Geometry: final body of the model. Coordinates: model frame, mm. Face numbers are marked on the shaded views. A direction names the side the tool comes from. Coordinates: 2 decimals unless noted, no trailing zeros. Loops run counter-clockwise (first coordinate to the right, second up) from the corner with the lowest first, then second, coordinate; pieces in that order, holes last. Notation, with made-up numbers: (40, 35) - (78, 35) arc R10 ccw to (78, 51) - close; hole circle Ø3 at (18, -31). An arc over 180 degrees is marked (long way). Answer in a Markdown table with one row per item.
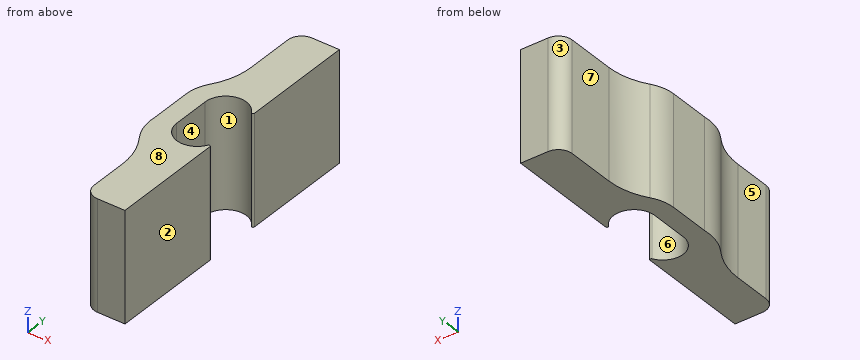
from build123d import *

# Parameters (mm, degrees)
F1_DEPTH = 8
F2_R     = 0.1
F3_R     = 1
F4_R     = 5


with BuildPart() as f1:
    # F0 (on Top) → F1 (new body)
    with BuildSketch(Plane.XY):
        with BuildLine():
            Line((0, -2.75), (0, 0))
            ThreePointArc((0, 0), (1.5, 1.5), (3, 0))
            Line((3, 0), (3, 9))
            Line((3, 9), (0, 9))
            Line((0, 9), (0, 2.4526771088))
            ThreePointArc((0, 2.4526771088), (-1.007800331, 1.4059027349), (-1.375, 0))
            Line((-1.375, 0), (-1.375, -3))
            ThreePointArc((-1.375, -3), (-1.1039614046, -4.7622217371), (0, -6.1622776602))
            Line((0, -6.1622776602), (0, -11.75))
            Line((0, -11.75), (3, -11.75))
            Line((3, -11.75), (3, -2.75))
            ThreePointArc((3, -2.75), (1.5, -4.25), (0, -2.75))
        make_face()
    extrude(amount=F1_DEPTH)

    # F2 (call 1 of 2: OpenCascade refuses the feature's edges together)
    f2_edges = [f1.edges().sort_by_distance(p)[0] for p in [
        (3, 0, 4),
    ]]
    fillet(f2_edges, radius=F2_R)

    # F2#2 (call 2 of 2)
    f2_2_edges = [f1.edges().sort_by_distance(p)[0] for p in [
        (3, -2.75, 4),
    ]]
    fillet(f2_2_edges, radius=F2_R)

    # F3
    f3_edges = [f1.edges().sort_by_distance(p)[0] for p in [
        (0, 9, 4),
        (0, -11.75, 4),
    ]]
    fillet(f3_edges, radius=F3_R)

    # F4
    f4_edges = [f1.edges().sort_by_distance(p)[0] for p in [
        (0, 2.452677, 4),
        (0, -6.162278, 4),
    ]]
    fillet(f4_edges, radius=F4_R)


solid = f1.part
(1) Cut plane B-B on x = 2.35. Output: boundary loops of the cut face in (y, z).
Verdict:
| item | result |
|---|---|
| outline | (-11.75, 0) - (-3.99, 0) - (-3.99, 8) - (-11.75, 8) - close; (1.24, 0) - (9, 0) - (9, 8) - (1.24, 8) - close |
(2) Access query for the marked faces 4, 5, 6, 7 and 8. Directions: +Z, -Z, +X, -X, +Y, -Y. A direction counts if a zero-diameter tool reaches every point of the face in a straight line with its end or side. Return the directions, or none.
Verdict:
| item | result |
|---|---|
| face 4 | +Z, -Z, +X |
| face 5 | +Z, -Z, -X, -Y |
| face 6 | +Z, -Z |
| face 7 | +Z, -Z, -X, +Y |
| face 8 | +Z, +X, -X, +Y, -Y |
(3) Ray query, probe 1 along X at (y, z) = (-1.75, 5.75) (3 decimals); probe 2 along Y at (x, z) = (1.85, 5); probe 3 along X at (y, z) = (5, 2.5). Return the intervals inside material, ascending.
Verdict:
| item | result |
|---|---|
| probe 1 | x = -1.375 to 0 |
| probe 2 | y = -11.75 to -4.21, 1.46 to 9 |
| probe 3 | x = 0 to 3 |
(4) Cut plane C-C on y = 6.75. Output: boundary loops of the cut face in (x, z), then the cut area to 3 significant figures.
Verdict:
| item | result |
|---|---|
| outline | (0, 0) - (3, 0) - (3, 8) - (0, 8) - close |
| area | 24.0 mm² |
(5) Pull-direction query (X, two-part tool) for the marked faces 1, 2 and 3; classes: pulls with the +X half, pulls with the -X half, needs draft (parallel to the pull), parting line crosses it, or undercut.
Verdict:
| item | result |
|---|---|
| face 1 | undercut |
| face 2 | pulls with the +X half |
| face 3 | pulls with the -X half |
(6) Cut plane D-D on x = -0.25. Output: boundary loops of the cut face in (y, z).
Verdict:
| item | result |
|---|---|
| outline | (-6.47, 0) - (2.88, 0) - (2.88, 8) - (-6.47, 8) - close |
(7) Cut plane A-A on y = -3.75. Output: boundary loops of the cut face in (x, z).
Verdict:
| item | result |
|---|---|
| outline | (-1.37, 0) - (0.38, 0) - (0.38, 8) - (-1.37, 8) - close; (2.62, 0) - (3, 0) - (3, 8) - (2.62, 8) - close |
(8) First-contact query: pin 1 Ø3.5 at (y, z) = (-1.5, 5.5) entering from -X; pin 2 Ø1.1 at (y, z) = (6.5, 4) entering from -X; pin 3 Ø3 at (y, z) = (-1.5, 5) entering from +X; pin 4 Ø1 at (x, y) = (2, -0.5) entering from -Z (1 decimal). Flat tips, straight axial feed; report the tip coordinate or a pass-through.
Verdict:
| item | result |
|---|---|
| pin 1 | stops at x = -1.39 |
| pin 2 | stops at x = 0 |
| pin 3 | stops at x = 0.02 |
| pin 4 | passes through |
